Could you check a few things on this model? Use its own coordinates, in mm. Face numbers are marked on the shaded views. A direction names the side the tool comes from. Give positions to 0.01 mm unless a question says otherwise; leave off trailing zeros. Write each loop counter-clockwise with the first axis right and the second up, starting at its lowest first coordinate (ties: lowest second). Pieces come first, ordered by that corner, then holes. Notation, with made-up numbers: M -9.5,89 L 26.5,89 A20 ccw 26.5,108 Z; hole C -18.5,53 d4. An arc over 180 degrees is marked long. One line per item, written item: value.
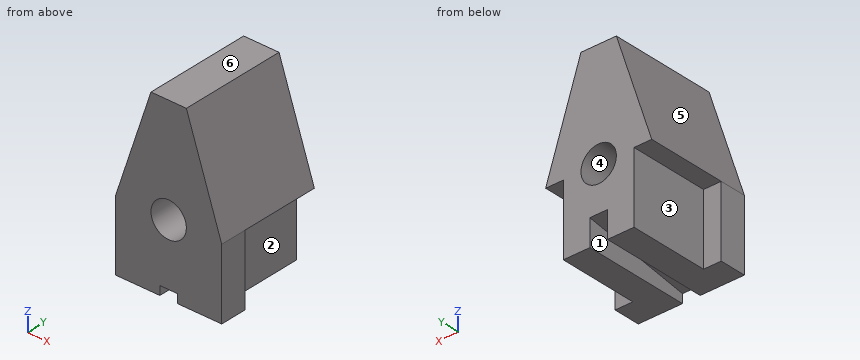
```python
from build123d import *

# Parameters (mm, degrees)
F0_R     = 10
F1_DEPTH = 60
F2_W     = 10
F2_H     = 40
F3_DEPTH = 45
F5_DEPTH = 5


with BuildPart() as f1:
    # F0 (on Front) → F1 (new body)
    with BuildSketch(Plane.XZ):
        Polygon((-30, 40), (-30, 0), (30, 0), (30, 40), (10, 100), (-10, 100), align=None)
        with Locations((0, 40)):
            Circle(F0_R, mode=Mode.SUBTRACT)
    extrude(amount=F1_DEPTH)

    # F2 (on face) → F3 (cut)
    with BuildSketch(Plane(origin=(0, 0, 0), x_dir=(-1, 0, 0), z_dir=(0, 1, 0))):
        with Locations((25, 20)):
            Rectangle(F2_W, F2_H)
        with Locations((-25, 20)):
            Rectangle(F2_W, F2_H)
    extrude(amount=-F3_DEPTH, mode=Mode.SUBTRACT)

    # F4 (on Right) → F5 (cut, symmetric)
    with BuildSketch(Plane.YZ):
        Polygon((-60, 5), (-60, 0), (-45, 0), (0, 0), (0, 15), align=None)
    extrude(amount=F5_DEPTH, both=True, mode=Mode.SUBTRACT)


solid = f1.part
```
1) I'm going to push flat-ended pins straight in: pin 1 (12 mm diameter, centred on y = -25, z = 71, fed in from -X); pin 2 (1 mm diameter, centred on y = -43.5, z = 46.5, fed in from +X); pin 3 (20 mm diameter, centred on y = -27, z = 18, fed in from -X). Where does each tip first touch, or does it pass through?
Outcome:
pin 1: stops at x = -21.67
pin 2: stops at x = 28
pin 3: stops at x = -20
2) If we section it at B-B, the plane y = -48: Write out the boundary of the cut face in (x, z), then the cut area to 3 significant figures.
Outcome:
outline: M -30,0 L -5,0 L -5,7 L 5,7 L 5,0 L 30,0 L 30,40 L 10,100 L -10,100 L -30,40 Z; hole C 0,40 d20
area: 4,420 mm^2
3) We'd pull the mould along X, two halves only. Please class the marked faces 4, 5 and 6: pulls with the +X half, pulls with the -X half, needs draft (parallel to the pull), parting line crosses it, or undercut.
Outcome:
face 4: undercut
face 5: pulls with the -X half
face 6: needs draft
4) On a 3-axis mill with a long thin cutter (end or side, diameter ignored), from which of +Z, -Z, +X, -X, +Y, -Y can I reach the whole of each face in a straight line? I mean the marked faces 1, 2 and 3. Say none if no direction works.
Outcome:
face 1: -Z, +Y
face 2: -Z, +X, +Y
face 3: -Z, -X, +Y
5) If we section it at A-A, the plane x = 0: Write out the boundary of the cut face in (y, z).
Outcome:
outline: M -60,5 L 0,15 L 0,30 L -60,30 Z; M -60,50 L 0,50 L 0,100 L -60,100 Z
6) If we section it at C-C, the plane z = 47: Write out the boundary of the cut face in (x, y), then the cut area to 3 significant figures.
Outcome:
outline: M -27.67,-60 L -7.14,-60 L -7.14,0 L -27.67,0 Z; M 7.14,-60 L 27.67,-60 L 27.67,0 L 7.14,0 Z
area: 2,460 mm^2
7) Please list where these lines run through material, in increasing order: L1, parallel to Z at x = 0, y = -14; L2, parallel to Z at x = 0, y = -38; L3, parallel to X at y = -35, z = 17.5. Write a range as from..to.
Outcome:
L1: z = 12.67..30, 50..100
L2: z = 8.67..30, 50..100
L3: x = -20..20
8) If we section it at D-D, the plane x = 24: Write out the boundary of the cut face in (y, z), then the cut area to 3 significant figures.
Outcome:
outline: M -60,0 L -45,0 L -45,40 L 0,40 L 0,58 L -60,58 Z
area: 1,680 mm^2
